```python
from build123d import *

# Parameters (mm, degrees)
F0_R      = 4.1
F1_DEPTH  = 12
F2_DEPTH  = 12
F4_DEPTH  = 3
F6_DEPTH  = 8
F7_DEPTH  = 9.5
F8_W      = 12
F8_H      = 2
F8_H_2    = 0.5
F9_DEPTH  = 25
F10_R     = 1
F11_R     = 0.5
F12_R     = 4.1
F13_DEPTH = 25
F14_DEPTH = 25


with BuildPart() as f1:
    # F0 (on Top) → F1 (new body)
    with BuildSketch(Plane.XY):
        with BuildLine():
            ThreePointArc((0, -6), (4.2426406871, -4.2426406871), (6, 0))
            ThreePointArc((6, 0), (4.2426406871, 4.2426406871), (0, 6))
            ThreePointArc((0, 6), (-4.2426406871, 4.2426406871), (-6, 0))
            ThreePointArc((-6, 0), (-4.2426406871, -4.2426406871), (0, -6))
        make_face()
        Circle(F0_R, mode=Mode.SUBTRACT)
    extrude(amount=F1_DEPTH)

    # F0 (on Top) → F2 (join)
    with BuildSketch(Plane.XY):
        with BuildLine():
            ThreePointArc((-6, 0), (-4.2426406871, 4.2426406871), (0, 6))
            Line((0, 6), (-6, 6))
            Line((-6, 6), (-6, 0))
        make_face()
        with BuildLine():
            Line((-6, -6), (0, -6))
            ThreePointArc((0, -6), (-4.2426406871, -4.2426406871), (-6, 0))
            Line((-6, 0), (-6, -6))
        make_face()
        Polygon((-6, -6), (-6, 0), (-6, 6), (-10.8, 6), (-10.8, -6), align=None)
    extrude(amount=F2_DEPTH)

    # F3 (on face) → F4 (cut)
    with BuildSketch(Plane.XY.offset(12)):
        Polygon((-5.6, -3), (-5.6, 0), (-5.6, 3), (-8.2, 3), (-8.2, -3), align=None)
    extrude(amount=F4_DEPTH, mode=Mode.SUBTRACT)

    # F5 (on face) → F6 (cut)
    with BuildSketch(Plane(origin=(-10.8, 0, 0), x_dir=(0, -1, 0), z_dir=(-1, 0, 0))):
        with BuildLine():
            ThreePointArc((0, 4.5), (1.0606601718, 4.9393398282), (1.5, 6))
            ThreePointArc((1.5, 6), (-1.0606601718, 7.0606601718), (0, 4.5))
        make_face()
    extrude(amount=-F6_DEPTH, mode=Mode.SUBTRACT)

    # F3 (on face) → F7 (cut)
    with BuildSketch(Plane.XY.offset(12)):
        Polygon((-5.6, -3), (-5.6, 0), (-5.6, 3), (-8.2, 3), (-8.2, -3), align=None)
    extrude(amount=-F7_DEPTH, mode=Mode.SUBTRACT)

    # F8 (on face) → F9 (cut)
    with BuildSketch(Plane(origin=(-10.8, 0, 0), x_dir=(0, -1, 0), z_dir=(-1, 0, 0))):
        with Locations((0, 11)):
            Rectangle(F8_W, F8_H)
        with Locations((0, 0.25)):
            Rectangle(F8_W, F8_H_2)
    extrude(amount=-F9_DEPTH, mode=Mode.SUBTRACT)

    # F10
    f10_edges = [f1.edges().sort_by_distance(p)[0] for p in [
        (-5.4, 6, 10),
        (-10.8, 0, 10),
        (-10.8, 6, 5.25),
        (-10.8, -6, 5.25),
    ]]
    fillet(f10_edges, radius=F10_R)

    # F11
    f11_edges = [f1.edges().sort_by_distance(p)[0] for p in [
        (-10.8, 0, 7.5),
        (-8.2, 0, 10),
        (-6.9, 3, 10),
        (-5.6, 0, 10),
        (-6.9, -3, 10),
        (-4.1, 0, 10),
        (-4.1, 0, 0.5),
    ]]
    fillet(f11_edges, radius=F11_R)

    # F12 (on face) → F13 (join)
    with BuildSketch(Plane(origin=(0, 0, 0.5), x_dir=(1, 0, 0), z_dir=(0, 0, -1))):
        Circle(F12_R)
    extrude(amount=-F13_DEPTH)

    # F14 (cut): a face of the model
    f14_faces = [f1.faces().sort_by_distance(p)[0] for p in [
        (0, 0, 0.5),
    ]]
    extrude(f14_faces, amount=-F14_DEPTH, mode=Mode.SUBTRACT)


solid = f1.part
```
Input: part model. Units: mm. Frame: model coordinates. A direction names the side the tool comes from. Coordinates: 2 decimals unless noted, no trailing zeros. Write each loop counter-clockwise with the first axis right and the second up, starting at its lowest first coordinate (ties: lowest second). Pieces come first, ordered by that corner, then holes. Notation, with made-up numbers: (27, -36.5) -> (84, -36.5) arc R24 ccw to (84, -24.5) -> close; hole circle Ø2 at (-28, -5). An arc over 180 degrees is marked (long way). Write each question's results on one line, items separated by ' | '.
Item 1: Section query A-A on z = 2.25. Return loops of the section in (x, y).
Conclusion:
outline: (-10.8, -5) arc R1 ccw to (-9.8, -6) -> (0, -6) arc R6 ccw to (0, 6) -> (-9.8, 6) arc R1 ccw to (-10.8, 5) -> close; hole circle Ø8.2 at (0, 0)
Item 2: Set-up query: faces 5 (the flat face through (-8.2, 0, 8)), 6 (the flat face through (-6, 0, 0.5)). Return all of +Z, -Z, +X, -X, +Y, -Y with unobstructed straight access to the full face (end or side cutting, diameter ignored); none if empty.
Conclusion:
face 5: +Z | face 6: -Z, +X, -X, +Y, -Y
Item 3: Pin query (flat end, axial travel): pin 1 Ø5 at (y, z) = (0, 6) entering from -X; pin 2 Ø3 at (y, z) = (-3, 4.5) entering from +X; pin 3 Ø2 at (x, z) = (3.5, 7.5) entering from +Y; pin 4 Ø1.5 at (x, y) = (3, -1) entering from +Z. Return the tip coordinate at first contact, or that it passes through.
Conclusion:
pin 1: stops at x = -10.8 | pin 2: stops at x = 5.81 | pin 3: stops at y = 5.45 | pin 4: passes through
Item 4: Material intervals for probe 1 along Y at (x, z) = (-9.55, 6); probe 2 along Z at (x, y) = (-8.85, 0); probe 3 along Y at (x, z) = (0, 3.5), sorted ascending.
Conclusion:
probe 1: y = -6 to -1.5, 1.5 to 6 | probe 2: z = 0.5 to 4.5, 7.5 to 10 | probe 3: y = -6 to -4.1, 4.1 to 6
Item 5: Mould query, pull axis X, two halves, no side actions, for faces 1 (the flat face through (-10.8, 0.1, 3.7)), 2 (the flat face through (-7, 0, 2.5)), 3 (the cylindrical face through (-4.831, 5.715, 9.699)), 4 (the cylindrical face through (3.91, -1.23, 5.19)). Classes: +X half, -X half, draft (parallel to the pull), parting line (faces both ways), or undercut.
Conclusion:
face 1: -X half | face 2: undercut | face 3: draft | face 4: undercut
Item 6: Section query B-B on y = -0.5. Count the separate pieces of the cut face and the enclosed holes in it, plus the area to 3 significant figures.
Conclusion:
separate pieces: 4 | enclosed holes: 0 | area: 50.0 mm^2
